Autodesk Inventor part; units mm, degrees
ref_plane "YZ Plane" through (0, 0, 0) normal (1, 0, 0) x (0, 1, 0)
ref_plane "XZ Plane" through (0, 0, 0) normal (0, 1, 0) x (-1, 0, 0)
ref_plane "XY Plane" through (0, 0, 0) normal (0, 0, 1) x (1, 0, 0)
sketch "Szkic1" plane through (0, 0, 0) normal (0, 1, 0) x (-1, 0, 0)
  line L0 (65, 0) -> (0, 0)
  line L1 (0, 0) -> (0, -120)
  line L2 (0, -120) -> (65, -120)
  line L3 (65, -120) -> (65, 0)
  dimension "d0" = 120
  dimension "d1" = 65
extrude "Gabaryt" add sketch "Szkic1" along normal blind 2
sketch "Szkic2" plane through (0, 0, 0) normal (0, 1, 0) x (1, 0, 0)
  line L0 (0, 0) -> (0, 120)
  line L1 (-65, 0) -> (0, 0)
  line L2 (-65, 120) -> (-65, 0)
  line L3 (0, 120) -> (-65, 120)
  line L4 (-65, 60) -> (0, 60)
  line L5 (-32.5, 120) -> (-32.5, 0)
  point P0 (-4, 4)
  point P1 (-61, 4)
  point P2 (-4, 116)
  point P3 (-61, 116)
  dimension "d4" = 4
  dimension "d5" = 4
hole "Otwory montażowe" at (-4, 0, -4) at (-61, 0, -4) at (-61, 0, -116) at (-4, 0, -116) direction (0, 1, 0) diameter 2.6 end through all counterbore diameter 4.5 counterbore depth 1.5
fillet "Zaokrąglenie1" radius 3 4 edges at (0, 1, 0) (-65, 1, 0) (-65, 1, -120) (0, 1, -120)
equation "\"d0\" = podstawa_a"
equation "\"d1\" = podstawa_b"
equation "\"d2\" = podstawa_wys"
equation "\"d6\" = gniazdo_M2_D2"
equation "\"d8\" = gniazdo_M2_D1"
equation "\"d9\" = gniazdo_M2_glebokosc"
equation "\"d13\" = podstawa_zaokraglenie"
equation "\"podstawa_a\" = 120"
equation "\"podstawa_b\" = 65"
equation "\"podstawa_wys\" = 2"
equation "\"podstawa_otwory_montazowe_poz_y\" = 4"
equation "\"podstawa_otwory_montazowe_poz_x\" = 4"
equation "\"gniazdo_M2_D1\" = 4.5"
equation "\"gniazdo_M2_glebokosc\" = 1.5"
equation "\"gniazdo_M2_D2\" = 2.6"
equation "\"obudowa_b\" = 65"
equation "\"obudowa_wys\" = 36"
equation "\"obudowa_grubosc\" = 2"
equation "\"obudowa_prowadnica_odsuniecie\" = 2"
equation "\"obudowa_prowadnica_grubosc\" = 2"
equation "\"obudowa_kontrolki_a\" = 38"
equation "\"obudowa_prowadnica_wys\" = 19"
equation "\"obudowa_otwory_montazowe_poz_y\" = 4"
equation "\"obudowa_otwory_montazowe_poz_x\" = 4"
equation "\"obudowa_otwory_montazowe_material_y\" = 8"
equation "\"obudowa_otwory_montazowe_material_x\" = 8"
equation "\"insert_D\" = 2.4"
equation "\"insert_glebokosc\" = 5.5"
equation "\"obudowa_zaokraglenie\" = 3"
equation "\"podstawa_zaokraglenie\" = 3"
equation "\"obudowa_otwory_io_wys\" = 15"
equation "\"obudowa_otwory_io_D\" = 15"
equation "\"obudowa_otwory_io1_wys\" = 15"
equation "\"obudowa_otwory_io1_D\" = 11.5"
equation "\"obudowa_otwory_io2_wys\" = 15"
equation "\"obudowa_otwory_io2_D\" = 11.5"
equation "\"obudowa_otwory_pot_D\" = 8"
equation "\"input_b\" = 14.4"
equation "\"input_wys\" = 11"
equation "\"input_a\" = 9"
properties part number "podstawa" material "Tworzywo sztuczne PET"
Build history of the part. All positions in model axes, mm. A direction names the side the tool comes from. Give positions to 0.01 mm unless a question says otherwise; leave off trailing zeros. Return JSON: item names as keys, results as strings.
Q1. Wall check: probe 1 along X at (y, z) = (1.9, -116); probe 2 along Z at (x, y) = (-4, 0.55); probe 3 along Z at (x, y) = (-61, 1.8). Give the ranges that are in metal, low to high. Write a range as from..to.
Answer list:
{"probe 1": "x = -65..-62.3, -59.7..-5.3, -2.7..0", "probe 2": "z = -120..-118.25, -113.75..-6.25, -1.75..0", "probe 3": "z = -120..-117.3, -114.7..-5.3, -2.7..0"}
Q2. 3-axis set-ups, long thin cutter, end or side, ignore diameter. For faces 5 (the face through (-60.5, 1.8, -117.2)), 6 (the face through (-3.14, 0.76, -118.08)): which of +Z, -Z, +X, -X, +Y, -Y reach the whole face in a straight line?
Answer list:
{"face 5": "+Y, -Y", "face 6": "-Y"}
Q3. Flat gauge pin, fed straight in: pin 1 (3.5 mm diameter, centred on x = -61, z = -4, fed in from -Y). Where does the tip first touch, or does it go through?
Answer list:
{"pin 1": "stops at y = 1.5"}
Q4. Two-plate mould, pull along X, no slides. Class faces 1 (the face through (-2.5, 1.5, -116)), 2 (the face through (-32, 0, -59)), 3 (the face through (-61, 1.5, -5.5)), 4 (the face through (-0.9, 1.01, -0.86)): pulls with the +X half, pulls with the -X half, needs draft (parallel to the pull), parting line crosses it, or undercut.
Answer list:
{"face 1": "undercut", "face 2": "needs draft", "face 3": "undercut", "face 4": "pulls with the +X half"}
